Source: CAD feature listing. Evaluate the final solid. Frame: model axes, mm. Face numbers are marked on the shaded views. Round coordinates to 2 decimals unless told otherwise and drop trailing zeros. Write each loop counter-clockwise with the first axis right and the second up, starting at its lowest first coordinate (ties: lowest second). Pieces come first, ordered by that corner, then holes. Notation, with made-up numbers: M -1.75,2 L 22.25,2 A27 ccw 22.25,29 Z; hole C 44.25,29 d7. An arc over 180 degrees is marked long. Use a Markdown table: item, result.
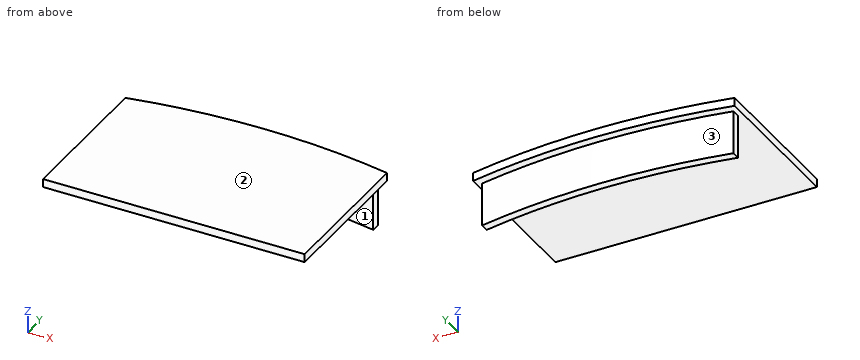
```python
from build123d import *

# Parameters (mm, degrees)
F1_DEPTH = 19
F3_DEPTH = 100


# Not quite as in the source:
# - a feature of the source that left no trace in its solid (it failed there, or was rolled back) is left out


with BuildPart() as f1:
    # F0 (on Top) → F1 (new body)
    with BuildSketch(Plane.XY):
        with BuildLine():
            Line((-300, -175), (300, -175))
            Line((300, -175), (300, 175))
            ThreePointArc((300, 175), (0, 204.3093674254), (-300, 175))
            Line((-300, 175), (-300, -175))
        make_face()
    extrude(amount=F1_DEPTH)

    # F2 (on face) → F3 (join)
    with BuildSketch(Plane(origin=(0, 0, 0), x_dir=(1, 0, 0), z_dir=(0, 0, -1))):
        with BuildLine():
            Line((-288, -138.6273926478), (-288, -157.9772163868))
            ThreePointArc((-288, -157.9772163868), (0, -185.3093674254), (288, -157.9772163868))
            Line((288, -157.9772163868), (288, -138.6273926478))
            ThreePointArc((288, -138.6273926478), (0, -166.3093674254), (-288, -138.6273926478))
        make_face()
    extrude(amount=F3_DEPTH)


solid = f1.part
```
Q1. Line query: L1, parallel to Z at x = -168, y = -50; L2, parallel to Y at x = 174.5, z = -60; L3, parallel to Y at x = 225.5, z = -34. Output: solid intervals per line, ascending.
Results are:
| item | result |
|---|---|
| L1 | 0 to 19 |
| L2 | 156.21 to 175.33 |
| L3 | 149.4 to 168.61 |
Q2. Section C-C on y = 57. Return loops of the section in (x, z).
Results are:
| item | result |
|---|---|
| outline | M -300,0 L 300,0 L 300,19 L -300,19 Z |
Q3. Mould query, pull axis X, two halves, no side actions, for the marked faces 1, 2 and 3. Classes: +X half, -X half, draft (parallel to the pull), parting line (faces both ways), or undercut.
Results are:
| item | result |
|---|---|
| face 1 | undercut |
| face 2 | draft |
| face 3 | parting line |
Q4. First-contact query: pin 1 Ø6 at (y, z) = (158.5, -40) entering from -X; pin 2 Ø1 at (x, y) = (-1, 123.5) entering from -Z; pin 3 Ø21.5 at (y, z) = (145.5, -26.5) entering from +X. Flat tips, straight axial feed; report the tip coordinate or a pass-through.
Results are:
| item | result |
|---|---|
| pin 1 | x = -288 |
| pin 2 | z = 0 |
| pin 3 | x = 288 |
Q5. Section B-B on z = -82.5. Return loops of the section in (x, y).
Results are:
| item | result |
|---|---|
| outline | M -288,138.63 A1512 cw 288,138.63 L 288,157.98 A1531 ccw -288,157.98 Z |
Q6. Section A-A on x = -84.5. Return loops of the section in (y, z).
Results are:
| item | result |
|---|---|
| outline | M -175,0 L 163.95,0 L 163.95,-100 L 182.98,-100 L 182.98,0 L 202,0 L 202,19 L -175,19 Z |
Q7. Section D-D on x = -197.5. Return loops of the section in (y, z), plus the area to 3 significant figures.
Results are:
| item | result |
|---|---|
| outline | M -175,0 L 153.35,0 L 153.35,-100 L 172.52,-100 L 172.52,0 L 191.68,0 L 191.68,19 L -175,19 Z |
| area | 8,880 mm^2 |
